```python
from build123d import *

# Parameters (mm, degrees)
F0_R      = 7
F1_DEPTH  = 16.75
F2_R      = 7
F3_DEPTH  = 12
F4_R      = 22.5
F5_DEPTH  = 6
F6_SIZE   = 1.5
F7_R      = 21
F8_DEPTH  = 24
F9_SIZE   = 1.5
F10_R     = 12.5
F11_DEPTH = 63.501
F12_R     = 42
F12_R_2   = 12.5
F13_DEPTH = 18
F14_R     = 7.5
F14_R_2   = 4.25
F15_DEPTH = 2
F16_DEPTH = 9


with BuildPart() as f1:
    # F0 (on Front) → F1 (new body, symmetric)
    with BuildSketch(Plane.XZ):
        with BuildLine():
            Line((-37.5, -47.5), (37.5, -47.5))
            ThreePointArc((37.5, -47.5), (44.5710678119, -44.5710678119), (47.5, -37.5))
            Line((47.5, -37.5), (47.5, 37.5))
            ThreePointArc((47.5, 37.5), (44.5710678119, 44.5710678119), (37.5, 47.5))
            Line((37.5, 47.5), (-37.5, 47.5))
            ThreePointArc((-37.5, 47.5), (-44.5710678119, 44.5710678119), (-47.5, 37.5))
            Line((-47.5, 37.5), (-47.5, -37.5))
            ThreePointArc((-47.5, -37.5), (-44.5710678119, -44.5710678119), (-37.5, -47.5))
        make_face()
        with Locations((-36, -36)):
            Circle(F0_R, mode=Mode.SUBTRACT)
        with Locations((36, -36)):
            Circle(F0_R, mode=Mode.SUBTRACT)
        with Locations((-36, 36)):
            Circle(F0_R, mode=Mode.SUBTRACT)
        with Locations((36, 36)):
            Circle(F0_R, mode=Mode.SUBTRACT)
    extrude(amount=F1_DEPTH, both=True)

    # F2 (on face) → F3 (cut)
    with BuildSketch(Plane.XZ.offset(16.75)):
        with BuildLine():
            Line((22, -42), (22, -47.5))
            Line((22, -47.5), (37.5, -47.5))
            ThreePointArc((37.5, -47.5), (44.5710678119, -44.5710678119), (47.5, -37.5))
            Line((47.5, -37.5), (47.5, -22))
            Line((47.5, -22), (42, -22))
            ThreePointArc((42, -22), (27.8578643763, -27.8578643763), (22, -42))
        make_face()
        with Locations((36, -36)):
            Circle(F2_R, mode=Mode.SUBTRACT)
        with BuildLine():
            Line((37.5, 47.5), (22, 47.5))
            Line((22, 47.5), (22, 42))
            ThreePointArc((22, 42), (27.8578643763, 27.8578643763), (42, 22))
            Line((42, 22), (47.5, 22))
            Line((47.5, 22), (47.5, 37.5))
            ThreePointArc((47.5, 37.5), (44.5710678119, 44.5710678119), (37.5, 47.5))
        make_face()
        with Locations((36, 36)):
            Circle(F2_R, mode=Mode.SUBTRACT)
        with BuildLine():
            Line((-47.5, 37.5), (-47.5, 22))
            Line((-47.5, 22), (-42, 22))
            ThreePointArc((-42, 22), (-27.8578643763, 27.8578643763), (-22, 42))
            Line((-22, 42), (-22, 47.5))
            Line((-22, 47.5), (-37.5, 47.5))
            ThreePointArc((-37.5, 47.5), (-44.5710678119, 44.5710678119), (-47.5, 37.5))
        make_face()
        with Locations((-36, 36)):
            Circle(F2_R, mode=Mode.SUBTRACT)
        with BuildLine():
            Line((-42, -22), (-47.5, -22))
            Line((-47.5, -22), (-47.5, -37.5))
            ThreePointArc((-47.5, -37.5), (-44.5710678119, -44.5710678119), (-37.5, -47.5))
            Line((-37.5, -47.5), (-22, -47.5))
            Line((-22, -47.5), (-22, -42))
            ThreePointArc((-22, -42), (-27.8578643763, -27.8578643763), (-42, -22))
        make_face()
        with Locations((-36, -36)):
            Circle(F2_R, mode=Mode.SUBTRACT)
    extrude(amount=-F3_DEPTH, mode=Mode.SUBTRACT)

    # F4 (on face) → F5 (join)
    with BuildSketch(Plane.XZ.offset(16.75)):
        Circle(F4_R)
    extrude(amount=F5_DEPTH)

    # F6
    f6_edges = [f1.edges().sort_by_distance(p)[0] for p in [
        (-22.5, -22.75, 0),
    ]]
    chamfer(f6_edges, length=F6_SIZE)

    # F7 (on face) → F8 (join)
    with BuildSketch(Plane.XZ.offset(22.75)):
        Circle(F7_R)
    extrude(amount=F8_DEPTH)

    # F9
    f9_edges = [f1.edges().sort_by_distance(p)[0] for p in [
        (-21, -46.75, 0),
    ]]
    chamfer(f9_edges, length=F9_SIZE)

    # F10 (on face) → F11 (cut, through all)
    with BuildSketch(Plane.XZ.offset(46.75)):
        Circle(F10_R)
    extrude(amount=-F11_DEPTH, mode=Mode.SUBTRACT)

    # F12 (on face) → F13 (cut)
    with BuildSketch(Plane(origin=(0, 16.75, 0), x_dir=(-1, 0, 0), z_dir=(0, 1, 0))):
        Circle(F12_R)
        Circle(F12_R_2, mode=Mode.SUBTRACT)
    extrude(amount=-F13_DEPTH, mode=Mode.SUBTRACT)

    # F14 (on face) → F15 (cut)
    with BuildSketch(Plane.YZ.offset(47.5)):
        with Locations((3.25, 7.547759451)):
            Circle(F14_R)
        with Locations((3.25, 7.547759451)):
            Circle(F14_R_2, mode=Mode.SUBTRACT)
    extrude(amount=-F15_DEPTH, mode=Mode.SUBTRACT)

    # F16 (cut): a face of the model
    f16_faces = [f1.faces().sort_by_distance(p)[0] for p in [
        (47.5, 3.25, 7.547759451),
    ]]
    extrude(f16_faces, amount=-F16_DEPTH, mode=Mode.SUBTRACT)


solid = f1.part
```
Input: part model. Units: mm. Frame: model coordinates. A direction names the side the tool comes from. Give positions to 0.01 mm unless a question says otherwise; leave off trailing zeros. Write each loop counter-clockwise with the first axis right and the second up, starting at its lowest first coordinate (ties: lowest second). Pieces come first, ordered by that corner, then holes. Notation, with made-up numbers: (38, 24.5) - (52, 24.5) arc R28 ccw to (52, 56.5) - close; hole circle Ø2 at (13.25, -9.75). An arc over 180 degrees is marked (long way). Write item = value, one per line. Start each with the question number.
1) Cut plane D-D (y = -3). Return loops of the section in (x, z), and give its area (3 significant figures).
2) Reachability of faces 1 (the face through (43.517, 2.697, 11.762)), 2 (the face through (-9, -1.25, 10)), 3 (the face through (22, -11, 45)) from +Z, -Z, +X, -X, +Y, -Y: full face, straight path, thin tool, end or side. Return the list, or none.
3) Cut plane C-C (x = 0). Return loops of the section in (y, z).
4) Pin query (flat end, axial travel): pin 1 (4.5 mm diameter, centred on x = 44, y = -12.5, fed in from +Z); pin 2 (4.5 mm diameter, centred on y = 4.5, z = 6.5, fed in from +X); pin 3 (22.5 mm diameter, centred on x = 36, z = -36, fed in from -Y). Return the tip coordinate at first contact, or that it passes through.
5) Cut plane A-A (x = 36). Return loops of the section in (y, z), and give its area (3 significant figures).
6) Cut plane B-B (z = -36). Return loops of the section in (x, y), and give its area (3 significant figures).
7) Draft query along Z for faces 4 (the face through (-40.06, 7.88, 12.62)), 5 (the face through (-45, -11, 22)), 6 (the face through (20.03, -33.84, 6.31)), 7 (the face through (-29, -4.75, 32)). Return one class per face: pulls with the +Z half, pulls with the -Z half, needs draft (parallel to the pull), parting line crosses it, or undercut.
8) Material intervals for L1, parallel to Z at x = 42.15, y = 3.25; L2, parallel to Z at x = -36, y = 8; L3, parallel to Z at x = 0, y = -19, sorted ascending. Write a range as [from, to].
Answers follow:
q1.outline = (-47.5, -37.5) arc R10 ccw to (-37.5, -47.5) - (37.5, -47.5) arc R10 ccw to (47.5, -37.5) - (47.5, 3.4) - (45.5, 3.4) - (45.5, 11.69) - (47.5, 11.69) - (47.5, 37.5) arc R10 ccw to (37.5, 47.5) - (-37.5, 47.5) arc R10 ccw to (-47.5, 37.5) - close; hole circle Ø14 at (-36, -36); hole circle Ø14 at (-36, 36); hole circle Ø25 at (0, 0); hole circle Ø14 at (36, -36); hole circle Ø14 at (36, 36)
q1.area = 7,820 mm^2
q2.face_1 = +X
q2.face_2 = +Y
q2.face_3 = +Z, +X, -Y
q3.outline = (-46.75, -19.5) - (-45.25, -21) - (-22.75, -21) - (-21.25, -22.5) - (-16.75, -22.5) - (-16.75, -47.5) - (16.75, -47.5) - (16.75, -42) - (-1.25, -42) - (-1.25, -12.5) - (-46.75, -12.5) - close; (-46.75, 12.5) - (-1.25, 12.5) - (-1.25, 42) - (16.75, 42) - (16.75, 47.5) - (-16.75, 47.5) - (-16.75, 22.5) - (-21.25, 22.5) - (-22.75, 21) - (-45.25, 21) - (-46.75, 19.5) - close
q4.pin_1 = 22
q4.pin_2 = -41.08
q4.pin_3 = -4.75
q5.outline = (-16.75, -22.92) - (-4.75, -22.92) - (-4.75, -29) - (16.75, -29) - (16.75, -21.63) - (-1.25, -21.63) - (-1.25, 21.63) - (16.75, 21.63) - (16.75, 29) - (-4.75, 29) - (-4.75, 22.92) - (-16.75, 22.92) - close; (-4.75, -47.5) - (16.75, -47.5) - (16.75, -43) - (-4.75, -43) - close; (-4.75, 43) - (16.75, 43) - (16.75, 47.5) - (-4.75, 47.5) - close
q5.area = 1,210 mm^2
q6.outline = (-47.5, -4.75) - (-43, -4.75) - (-43, 16.75) - (-47.5, 16.75) - close; (-29, -4.75) - (-22.92, -4.75) - (-22.92, -16.75) - (22.92, -16.75) - (22.92, -4.75) - (29, -4.75) - (29, 16.75) - (21.63, 16.75) - (21.63, -1.25) - (-21.63, -1.25) - (-21.63, 16.75) - (-29, 16.75) - close; (43, -4.75) - (47.5, -4.75) - (47.5, 16.75) - (43, 16.75) - close
q6.area = 1,210 mm^2
q7.face_4 = undercut
q7.face_5 = pulls with the +Z half
q7.face_6 = parting line crosses it
q7.face_7 = needs draft
q8.L1 = [-46.35, -39.34], [-32.66, 3.3], [11.8, 32.66], [39.34, 46.35]
q8.L2 = [-47.5, -43], [-29, -21.63], [21.63, 29], [43, 47.5]
q8.L3 = [-22.5, -12.5], [12.5, 22.5]
